Check sheet for the modelled part. Datum: model origin and axes. Units: mm. Give positions to 0.01 mm unless a question says otherwise; leave off trailing zeros. Write each loop counter-clockwise with the first axis right and the second up, starting at its lowest first coordinate (ties: lowest second). Pieces come first, ordered by that corner, then holes. Notation, with made-up numbers: M -40,23 L -18,23 A19 ccw -18,58 Z; hole C 32.25,72 d11. An arc over 180 degrees is marked long. Use CSV: the item, a comma, the result in double quotes. Start each with the question number.
1. Scan lines: line 1 (Z direction, x = -15, y = 16); line 2 (Z direction, x = 7.5, y = 1); line 3 (X direction, y = -1.5, z = 22). Record each from-to range of solid material in increasing order.
2. Depth check by flat-ended pin: P1, Ø1.5, axis at x = 10.5, z = 15, coming from the -Y side; P2, Ø1.5, axis at x = -17.5, y = 18, coming from the +Z side; P3, Ø3, axis at x = 7.5, z = 30, coming from the +Y side; P4, Ø6, axis at y = -12.5, z = 19, coming from the -X side. Enter the tip coordinate at first touch or a pass-through.
3. Cross-section at A-A, the plane x = -19. Enter the section's corners in (y, z), and give its area (3 significant figures).
4. Cross-section at B-B, the plane y = 8.5. Enter the section's corners in (x, z).
Solid Edge part; units mm, degrees
sketch "Sketch1" plane through (0, 0, 0) normal (0, 0, 1) x (1, 0, 0)
  line L0 (-25, -25) -> (25, -25)
  line L1 (25, -25) -> (25, 25)
  line L2 (25, 25) -> (-25, 25)
  line L3 (-25, 25) -> (-25, -25)
extrude "Protrusion1" add sketch "Sketch1" along normal blind 44.9981
sketch "Sketch2" plane through (0, 0, 0) normal (1, 0, 0) x (0, 1, 0)
  line L0 (-25, 0) -> (0, 35.3538)
extrude "ExtrudedCutout_1" cut sketch "Sketch2" against normal blind 70.8899 material side at (0, -12.5408, 17.7058)
sketch "Sketch3" plane through (0, 0, 0) normal (1, 0, 0) x (0, 1, 0)
  line L0 (-25, 0) -> (0, 35.3538)
extrude "ExtrudedCutout_2" cut sketch "Sketch3" along normal blind 62.8041 material side at (0, -12.5408, 17.7058)
pattern_circular "Pattern1" count 4 over 360 about axis through (0, 0, 0) along (0, 0, -1) of "ExtrudedCutout_2", "ExtrudedCutout_1"
Worked answers:
1,line 1,"z = 0 to 12.73"
1,line 2,"z = 0 to 24.75"
1,line 3,"x = -9.44 to 9.44"
2,P1,"stops at y = -14.92"
2,P2,"stops at z = 10.91"
2,P3,"passes through"
2,P4,"stops at x = -13.69"
3,outline,"M -25,0 L 25,0 L 19,8.48 L -19,8.48 Z"
3,area,"373 mm^2"
4,outline,"M -25,0 L 25,0 L 8.5,23.33 L -8.5,23.33 Z"
